The listing builds one solid part. Answer for the finished solid, in the listing's coordinates (mm). A direction names the side the tool comes from. Round coordinates to 2 decimals unless told otherwise and drop trailing zeros. Write each loop counter-clockwise with the first axis right and the second up, starting at its lowest first coordinate (ties: lowest second). Pieces come first, ordered by that corner, then holes. Notation, with made-up numbers: (59, 16.25) - (91, 16.25) arc R25 ccw to (91, 31.25) - close; hole circle Ø9 at (-18.75, 88). An arc over 180 degrees is marked (long way). Answer as CSV lines item,"result". Start each with the question number.
Item 1: A cutting plane is placed at D-D on z = 53.5. Determine the outline of the cut face in (x, y), and give its area (3 significant figures).
Item 2: Which of the six approach directions +Z, -Z, +X, -X, +Y, -Y give full straight-line access (tool end or side, diameter ignored) to faces 4 (the flat face through (13, -15.12, 20)), 5 (the flat face through (-7, 0, 40)), 6 (the cylindrical face through (27.87, 25.75, 16.55)), 7 (the flat face through (26, 38.42, 18))?
Item 3: Flat-ended cylindrical pins translate along their axes: pin 1 (5 mm diameter, centred on x = -1.5, y = 26.5, fed in from +Z); pin 2 (5 mm diameter, centred on y = 13.5, z = 12.5, fed in from -X); pin 3 (8 mm diameter, centred on y = 20.5, z = 10.5, fed in from +X). Find the tip coordinate at first contact, or state that the pin passes through.
Item 4: A cutting plane is placed at B-B on x = 0. Determine the outline of the cut face in (y, z), and give its area (3 significant figures).
Item 5: A cutting plane is placed at C-C on y = 25. Determine the outline of the cut face in (x, z).
Item 6: For a pull along X with two mould halves and no side action, classify faces 1 (the flat face through (16, 38.42, 18)), 2 (the cylindrical face through (6.81, 25.75, 14.17)), 3 (the flat face through (37.233, -1, 20)) as pulls with the +X half, pulls with the -X half, needs draft (parallel to the pull), parting line crosses it, or undercut.
Item 7: Straight lines are drawn through the part: line 1 along X through (y, z) = (24, 18.5); line 2 along Y through (x, z) = (1, 5); line 3 along Z through (x, y) = (-20, -11). For each, find the intervals that lie inside material, in ascending order. Write a range as [from, to].
Item 8: A cutting plane is placed at A-A on z = 30.5. Determine the outline of the cut face in (x, y).
```python
from build123d import *

# Parameters (mm, degrees)
F1_DEPTH = 70
F2_DEPTH = 40
F3_R     = 3
F4_R     = 2.5
F5_DEPTH = 25


with BuildPart() as f1:
    # F0 (on Top) → F1 (new body)
    with BuildSketch(Plane.XY):
        with BuildLine():
            ThreePointArc((-16.9023339674, 0), (-19.8312661555, 7.0710678119), (-26.9023339674, 10))
            Line((-26.9023339674, 10), (-26.9023339674, 5.8191100826))
            ThreePointArc((-26.9023339674, 5.8191100826), (-22.7876017675, 4.1147321999), (-21.0832238848, 0))
            ThreePointArc((-21.0832238848, 0), (-22.7876017675, -4.1147321999), (-26.9023339674, -5.8191100826))
            Line((-26.9023339674, -5.8191100826), (-26.9023339674, -10))
            ThreePointArc((-26.9023339674, -10), (-19.8312661555, -7.0710678119), (-16.9023339674, 0))
        make_face()
        with BuildLine():
            Line((-26.9023339674, 5.8191100826), (-26.9023339674, 10))
            ThreePointArc((-26.9023339674, 10), (-36.9023339674, 0), (-26.9023339674, -10))
            Line((-26.9023339674, -10), (-26.9023339674, -5.8191100826))
            ThreePointArc((-26.9023339674, -5.8191100826), (-32.7214440499, 0), (-26.9023339674, 5.8191100826))
        make_face()
    extrude(amount=F1_DEPTH)

    # F0 (on Top) → F2 (join)
    with BuildSketch(Plane.XY):
        with BuildLine():
            Line((37.2332856059, 13.4202644998), (21.7927563936, 13.4202644998))
            Line((21.7927563936, 13.4202644998), (-8.6679077107, 13.4202644998))
            ThreePointArc((-8.6679077107, 13.4202644998), (-5.391446413, 7.0625432229), (-4.261711181, 0))
            ThreePointArc((-4.261711181, 0), (-5.7584541043, -8.0953162068), (-10.0507873126, -15.1202901922))
            Line((-10.0507873126, -15.1202901922), (37.2332856059, -15.1202901922))
            Line((37.2332856059, -15.1202901922), (37.2332856059, 13.4202644998))
        make_face()
        with BuildLine():
            ThreePointArc((-4.261711181, 0), (-5.391446413, 7.0625432229), (-8.6679077107, 13.4202644998))
            Line((-8.6679077107, 13.4202644998), (-26.9023339674, 13.4202644998))
            Line((-26.9023339674, 13.4202644998), (-26.9023339674, 10))
            ThreePointArc((-26.9023339674, 10), (-19.8312661555, 7.0710678119), (-16.9023339674, 0))
            ThreePointArc((-16.9023339674, 0), (-19.8312661555, -7.0710678119), (-26.9023339674, -10))
            Line((-26.9023339674, -10), (-26.9023339674, -15.1202901922))
            Line((-26.9023339674, -15.1202901922), (-10.0507873126, -15.1202901922))
            ThreePointArc((-10.0507873126, -15.1202901922), (-5.7584541043, -8.0953162068), (-4.261711181, 0))
        make_face()
        with BuildLine():
            Line((-26.9023339674, 13.4202644998), (-8.6679077107, 13.4202644998))
            ThreePointArc((-8.6679077107, 13.4202644998), (-12.4988940391, 17.468220241), (-17.2027000327, 20.4576367571))
            ThreePointArc((-17.2027000327, 20.4576367571), (-49.0989219749, -4.4619817321), (-10.0507873126, -15.1202901922))
            Line((-10.0507873126, -15.1202901922), (-26.9023339674, -15.1202901922))
            Line((-26.9023339674, -15.1202901922), (-26.9023339674, -10))
            ThreePointArc((-26.9023339674, -10), (-36.9023339674, 0), (-26.9023339674, 10))
            Line((-26.9023339674, 10), (-26.9023339674, 13.4202644998))
        make_face()
    extrude(amount=F2_DEPTH)

    # F3
    f3_edges = [f1.edges().sort_by_distance(p)[0] for p in [
        (-36.902334, 0, 40),
        (-16.902334, 0, 55),
        (-36.902334, 0, 70),
    ]]
    fillet(f3_edges, radius=F3_R)

    # F4 (on face) → F5 (join)
    with BuildSketch(Plane(origin=(0, 13.4202644998, 0), x_dir=(-1, 0, 0), z_dir=(0, 1, 0))):
        with Locations((-25.8841626346, 18.0686339736)):
            Circle(F4_R)
        with Locations((-15.9560106695, 18.0668439716)):
            Circle(F4_R)
        with Locations((-7.9592689872, 16.3908023387)):
            Circle(F4_R)
        with Locations((0, 14.6713265902)):
            Circle(F4_R)
    extrude(amount=F5_DEPTH)


solid = f1.part
```
Geometry says:
1,outline,"circle Ø20 at (-26.9, 0); hole circle Ø11.64 at (-26.9, 0)"
1,area,"208 mm^2"
2,face 4,"+Z, -Z, +X, -Y"
2,face 5,"+Z"
2,face 6,"+Y"
2,face 7,"+Z, -Z, +X, -X, +Y"
3,pin 1,"stops at z = 17.17"
3,pin 2,"stops at x = -46.69"
3,pin 3,"stops at x = 9.59"
4,outline,"(-15.12, 0) - (13.42, 0) - (13.42, 12.17) - (38.42, 12.17) - (38.42, 17.17) - (13.42, 17.17) - (13.42, 40) - (-15.12, 40) - close"
4,area,"1,270 mm^2"
5,outline,"circle Ø5 at (0, 14.67); circle Ø5 at (7.96, 16.39); circle Ø5 at (15.96, 18.07); circle Ø5 at (25.88, 18.07)"
6,face 1,"needs draft"
6,face 2,"undercut"
6,face 3,"pulls with the +X half"
7,line 1,"x = [6.62, 9.3], [13.49, 18.42], [23.42, 28.35]"
7,line 2,"y = [-15.12, 13.42]"
7,line 3,"z = [0, 40]"
8,outline,"(-10.05, -15.12) - (37.23, -15.12) - (37.23, 13.42) - (-8.67, 13.42) arc R22.64 ccw (long way) to start; hole circle Ø11.64 at (-26.9, 0)"
